from build123d import *

# Parameters (mm, degrees)
SKETCH_R     = 1
PAD_DEPTH    = 4
POCKET_DEPTH = 0.5


with BuildPart() as part:
    # Sketch → Pad (new body)
    with BuildSketch(Plane(origin=(43, -2, 9), x_dir=(1, 0, 0), z_dir=(0, 1, 0))):
        with BuildLine():
            ThreePointArc((-0.223332, 3.993761), (-3.918859, -0.801586), (1.362808, -3.760685))
            ThreePointArc((1.362808, -3.760685), (33.201741, 2.472732), (62.334, 16.751548))
            ThreePointArc((62.334, 16.751548), (62.792415, 22.863986), (56.693532, 22.25106))
            ThreePointArc((-0.223332, 3.993761), (29.431262, 9.393393), (56.693532, 22.25106))
        make_face()
        Circle(SKETCH_R, mode=Mode.SUBTRACT)
        with Locations((60, 20)):
            Circle(SKETCH_R, mode=Mode.SUBTRACT)
    extrude(amount=PAD_DEPTH)

    # Sketch001 → Pocket (cut)
    with BuildSketch(Plane(origin=(43, 2, 9), x_dir=(1, 0, 0), z_dir=(0, 1, 0))):
        with BuildLine():
            ThreePointArc((4.422958, -1.803146), (31.876892, 3.906972), (57.301864, 15.734682))
            ThreePointArc((57.301864, 15.734682), (57.948359, 18.488233), (55.194808, 19.134728))
            ThreePointArc((4.063939, 2.180709), (30.609778, 7.70096), (55.194808, 19.134728))
            ThreePointArc((4.063939, 2.180709), (2.251525, 0.009273), (4.422958, -1.803146))
        make_face()
    extrude(amount=-POCKET_DEPTH, mode=Mode.SUBTRACT)


solid = part.part
The listing builds one solid part. Answer for the finished solid, in the listing's coordinates (mm). A direction names the side the tool comes from. Round coordinates to 2 decimals unless told otherwise and drop trailing zeros. Write each loop counter-clockwise with the first axis right and the second up, starting at its lowest first coordinate (ties: lowest second). Pieces come first, ordered by that corner, then holes. Notation, with made-up numbers: M 79.5,-21 L 118.5,-21 A34 cw 118.5,13 Z; hole C -36,5.25 d9. An arc over 180 degrees is marked long. Write each question's results on one line, items separated by ' | '. Start each with the question number.
Item 1: A cutting plane is placed at A-A on y = -0.65. Write down the section's boundary in (x, z).
Item 2: For faces 4 (the face through (74.503, 1.754, 5.216)), 5 (the face through (44, 0, 9)), determine the directions among +Z, -Z, +X, -X, +Y, -Y from which every point of the face is accessible in a straight line to the end or side of a thin tool.
Item 3: For a pull along X with two mould halves and no side action, classify faces 1 (the face through (73.248, 1.754, 1.418)), 2 (the face through (73, 2, 1)), 3 (the face through (105.862, -0.028, -13.795)) as pulls with the +X half, pulls with the -X half, needs draft (parallel to the pull), parting line crosses it, or undercut.
Item 4: A cutting plane is placed at C-C on z = 9. Write down the section's boundary in (x, y), and give its area (3 significant figures).
Item 5: A cutting plane is placed at D-D on x = 94.5. Write down the section's boundary in (y, z).
Item 6: Straight lines are drawn through the part: L1, parallel to Z at x = 43, y = 1.1; L2, parallel to Y at x = 52.5, z = 7; L3, parallel to X at y = 0.7, z = -11. For each, find the intervals that lie inside material, in ascending order. Write a range as [from, to].
Item 7: A cutting plane is placed at B-B on x = 103. Write down the section's boundary in (y, z), and give its area (3 significant figures).
Item 8: Flat-ended cylindrical pins translate along their axes: pin 1 Ø1.5 at (x, y) = (53.5, -1.5) entering from +Z; pin 2 Ø2 at (y, z) = (0, -2) entering from +X; pin 3 Ø1.2 at (x, z) = (43, 9) entering from +Y. Find the tip coordinate at first contact, or state that the pin passes through.
Check sheet entries:
1) outline: M 42.78,5.01 A116 cw 99.69,-13.25 A4 ccw long 105.33,-7.75 A124 ccw 44.36,12.76 A4 ccw long Z; hole C 43,9 d2; hole C 103,-11 d2
2) face 4: +Y | face 5: +Y, -Y
3) face 1: undercut | face 2: needs draft | face 3: parting line crosses it
4) outline: M 39,-2 L 42,-2 L 42,2 L 39,2 Z; M 44,-2 L 67.9,-2 L 67.9,2 L 60.03,2 L 60.03,1.5 L 45.25,1.5 L 45.25,2 L 44,2 Z | area: 100 mm²
5) outline: M -2,-10.1 L 2,-10.1 L 2,-7.96 L 1.5,-7.96 L 1.5,-3.39 L 2,-3.39 L 2,-1.31 L -2,-1.31 Z
6) L1: [4.99, 8], [10, 13] | L2: [-2, 1.5] | L3: [96.04, 102], [104, 107]
7) outline: M -2,-15 L 2,-15 L 2,-12 L -2,-12 Z; M -2,-10 L 2,-10 L 2,-6.24 L -2,-6.24 Z | area: 27.1 mm²
8) pin 1: z = 11.95 | pin 2: x = 97.59 | pin 3: through
